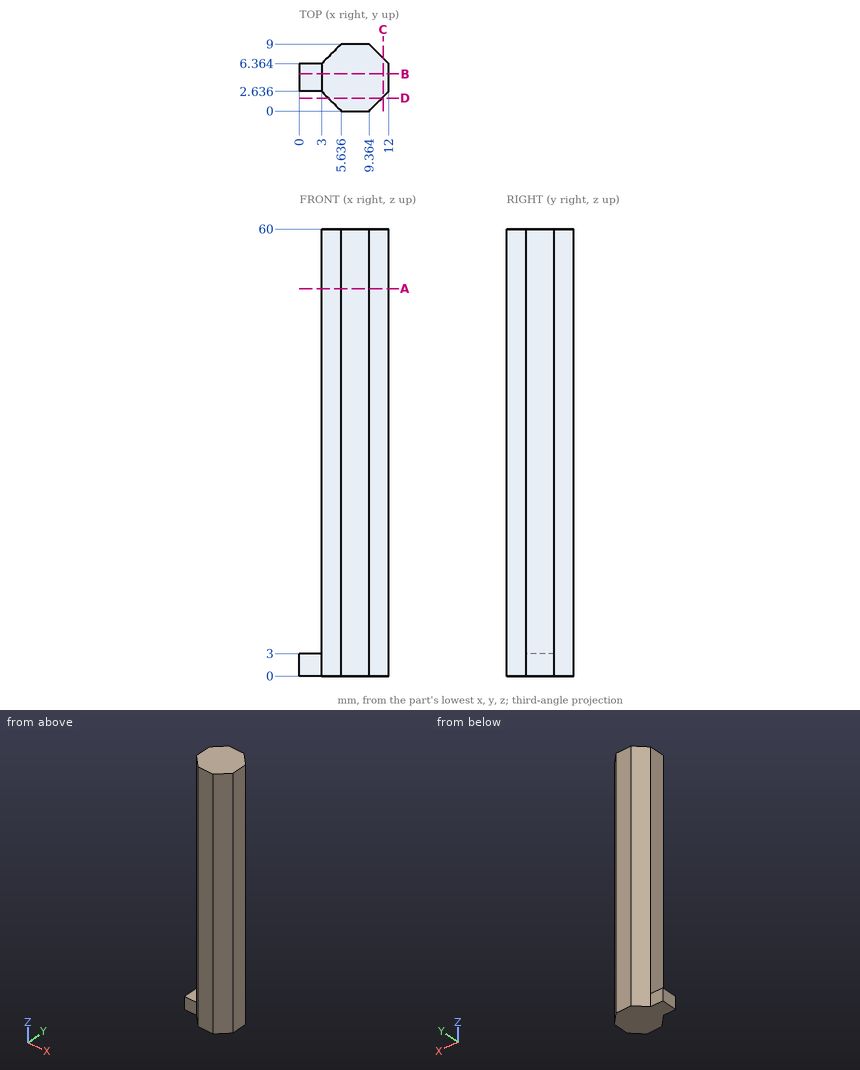
Input: dimensioned drawing with shaded views. Units: mm. Origin: part minimum x, y, z. Round coordinates to 2 decimals unless told otherwise and drop trailing zeros. Loops run counter-clockwise (first coordinate to the right, second up) from the corner with the lowest first, then second, coordinate; pieces in that order, holes last. Notation, with made-up numbers: (-5.75, -9.75) -> (42.25, -9.75) arc R14 ccw to (42.25, 17.25) -> close; hole circle Ø10 at (-16, 61.25). An arc over 180 degrees is marked (long way). Answer as a JSON object with one key per item and string values. Group by question number.
Q1. Section query C-C (x = 11.25). Output: boundary loops of the cut face in (y, z), plus the area to 3 significant figures.
Q2. Section query D-D (y = 1.75). Output: boundary loops of the cut face in (x, z), plus the area to 3 significant figures.
Q3. Section query B-B (y = 5). Output: boundary loops of the cut face in (x, z).
Q4. Ray query, line 1 (X direction, y = 5.75, z = 25); line 2 (Y direction, x = 3.25, z = 43); line 3 (X direction, y = 2.5, z = 26.5). Return the intervals inside material, ascending. Write a range as from..to.
Q5. Contact query for flat-ended pins moving along their axis: P1, Ø1.5, axis at x = 1, z = 1, coming from the -Y side; P2, Ø1.9, axis at y = 4.5, z = 39.5, coming from the -X side; P3, Ø1.5, axis at x = 2, z = 1, coming from the +Y side. Output: stop coordinate, or through.
Q6. Section query A-A (z = 52). Output: boundary loops of the cut face in (x, y), plus the area to 3 significant figures.
Completed:
{
 "1": {"outline": "(1.89, 0) -> (7.11, 0) -> (7.11, 60) -> (1.89, 60) -> close", "area": "314 mm²"},
 "2": {"outline": "(3.89, 0) -> (11.11, 0) -> (11.11, 60) -> (3.89, 60) -> close", "area": "434 mm²"},
 "3": {"outline": "(0, 0) -> (12, 0) -> (12, 60) -> (3, 60) -> (3, 3) -> (0, 3) -> close"},
 "4": {"line 1": "3..12", "line 2": "2.39..6.61", "line 3": "3.14..11.86"},
 "5": {"P1": "y = 2.64", "P2": "x = 3", "P3": "y = 6.36"},
 "6": {"outline": "(3, 2.64) -> (5.64, 0) -> (9.36, 0) -> (12, 2.64) -> (12, 6.36) -> (9.36, 9) -> (5.64, 9) -> (3, 6.36) -> close", "area": "67.1 mm²"}
}
